Build history of the part. All positions in model axes, mm. Face numbers are marked on the shaded views. A direction names the side the tool comes from. Give positions to 0.01 mm unless a question says otherwise; leave off trailing zeros. Loops run counter-clockwise (first coordinate to the right, second up) from the corner with the lowest first, then second, coordinate; pieces in that order, holes last.
1) Wall check: line 1 (X direction, y = 72, z = -6); line 2 (X direction, y = 9, z = 50); line 3 (Y direction, x = 0, z = 8). Give the ranges that are in metal, low to high.
2) Band-saw the part on C-C on y = 74.5. List the corners of the cut face in (x, z).
3) Two-plate mould, pull along Y, no slides. Class the marked faces 1, 2 and 3: +Y half, -Y half, draft (parallel to the pull), parting line (faces both ways), or undercut.
4) Band-saw the part on D-D on x = 21.5. List the corners of the cut face in (y, z), then the cut area to 3 significant figures.
5) Band-saw the part on A-A on x = 0. List the corners of the cut face in (y, z).
6) 3-axis set-ups, long thin cutter, end or side, ignore diameter. For the marked faces 4, 5, 6 and 7: which of +Z, -Z, +X, -X, +Y, -Y reach the whole face in a straight line?
7) Flat gauge pins, fed straight in: P1, Ø16.5, axis at x = -11, y = 73, coming from the +Z side; P2, Ø5, axis at x = -26, y = 39.5, coming from the +Z side; P3, Ø19.5, axis at x = 19, y = 30.5, coming from the -Z side. Where does each tip first touch, or does it go through?
8) Band-saw the part on B-B on z = -4. List the corners of the cut face in (x, y).
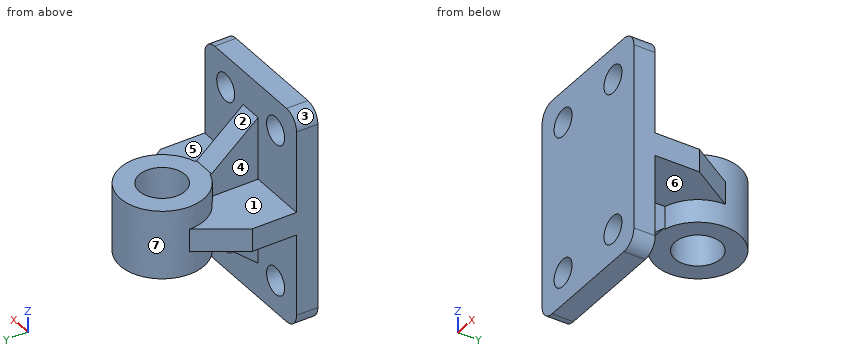
```python
from build123d import *

# Parameters (mm, degrees)
ESQUISSE1_W        = 92
ESQUISSE1_H        = 142
ESQUISSE1_R        = 9
BOSS_EXTRU_1_DEPTH = 14
CONG_1_R           = 10
ESQUISSE2_R        = 27.5
ESQUISSE2_R_2      = 15
BOSS_EXTRU_2_DEPTH = 22.5
BOSS_EXTRU_3_DEPTH = 7.5
NERVURE1_START     = -7.5
NERVURE1_DEPTH     = 15


with BuildPart() as part:
    # Esquisse1 → Boss.-Extru.1 (new body)
    with BuildSketch(Plane(origin=(0, 0, 0), x_dir=(1, 0, 0), z_dir=(0, 1, 0))):
        Rectangle(ESQUISSE1_W, ESQUISSE1_H)
        with Locations(Location((25, -50, 0), (0, 0, 270))):
            Circle(ESQUISSE1_R, mode=Mode.SUBTRACT)
        with Locations(Location((25, 50, 0), (0, 0, 90))):
            Circle(ESQUISSE1_R, mode=Mode.SUBTRACT)
        with Locations(Location((-25, -50, 0), (0, 0, 90))):
            Circle(ESQUISSE1_R, mode=Mode.SUBTRACT)
        with Locations(Location((-25, 50, 0), (0, 0, 270))):
            Circle(ESQUISSE1_R, mode=Mode.SUBTRACT)
    extrude(amount=BOSS_EXTRU_1_DEPTH)

    # Congé1
    cong_1_edges = [part.edges().sort_by_distance(p)[0] for p in [
        (46, 7, 71),
        (-46, 7, 71),
        (-46, 7, -71),
        (46, 7, -71),
    ]]
    fillet(cong_1_edges, radius=CONG_1_R)



with BuildPart() as body_2:
    # Esquisse2 → Boss.-Extru.2 (new, symmetric)
    with BuildSketch(Plane.XY):
        with Locations(Location((0, 72, 0), (0, 0, 180))):
            Circle(ESQUISSE2_R)
        with Locations(Location((0, 72, 0), (0, 0, 180))):
            Circle(ESQUISSE2_R_2, mode=Mode.SUBTRACT)
    extrude(amount=BOSS_EXTRU_2_DEPTH, both=True)


with BuildPart() as part_1:
    add(part.part)

    add(body_2.part)  # Boss.-Extru.3 merges body 2
    # Esquisse3 → Boss.-Extru.3 (add, symmetric)
    with BuildSketch(Plane.XY):
        with BuildLine():
            Line((46, 14), (46, 43))
            Line((46, 43), (27.5, 72))
            ThreePointArc((27.5, 72), (0, 44.5), (-27.5, 72))
            Line((-27.5, 72), (-46, 43))
            Line((-46, 43), (-46, 14))
            Line((-46, 14), (46, 14))
        make_face()
    extrude(amount=BOSS_EXTRU_3_DEPTH, both=True)

    # Nervure1: read off the stored shape, not the designer's step
    # Nervure1 outline → Nervure1 (add)
    with BuildSketch(Plane(origin=(0, 0, 0), x_dir=(0, 0, -1), z_dir=(1, 0, 0)).offset(NERVURE1_START)):
        Polygon((-22.5, 44.5), (-48.5, 14), (-7.5, 14), (-7.5, 45.542486889), (-22.5, 45.542486889), align=None)
    nervure1 = extrude(amount=NERVURE1_DEPTH)

    # Symétrie1: Nervure1 across plane
    add(nervure1.mirror(Plane.XY))


solid = part_1.part
```
Findings below:
1. line 1: x = -27.5 to -15, 15 to 27.5
1. line 2: x = -46 to -34, -16 to 16, 34 to 46
1. line 3: y = 0 to 57, 87 to 99.5
2. outline: (-27.39, -22.5) - (-14.79, -22.5) - (-14.79, 22.5) - (-27.39, 22.5) - close; (14.79, -22.5) - (27.39, -22.5) - (27.39, 22.5) - (14.79, 22.5) - close
3. face 1: undercut
3. face 2: +Y half
3. face 3: draft
4. outline: (0, -71) - (14, -71) - (14, -58.29) - (0, -58.29) - close; (0, -41.71) - (14, -41.71) - (14, -7.5) - (54.85, -7.5) - (54.85, -22.5) - (89.15, -22.5) - (89.15, 22.5) - (54.85, 22.5) - (54.85, 7.5) - (14, 7.5) - (14, 41.71) - (0, 41.71) - close; (0, 58.29) - (14, 58.29) - (14, 71) - (0, 71) - close
4. area: 3,680 mm2
5. outline: (0, -71) - (14, -71) - (14, -48.5) - (44.5, -22.5) - (57, -22.5) - (57, 22.5) - (44.5, 22.5) - (14, 48.5) - (14, 71) - (0, 71) - close; (87, -22.5) - (99.5, -22.5) - (99.5, 22.5) - (87, 22.5) - close
6. face 4: +Z, -X
6. face 5: +Z, +X
6. face 6: -Z, +X
6. face 7: none
7. P1: stops at z = 22.5
7. P2: stops at z = 7.5
7. P3: stops at z = -7.5
8. outline: (-46, 0) - (46, 0) - (46, 43) - (27.5, 72) arc R27.5 ccw to (-27.5, 72) - (-46, 43) - close; hole circle Ø30 at (0, 72)
